Design review of the part built by this model. Coordinates are the model's own, in mm. A direction names the side the tool comes from. Round coordinates to 2 decimals unless told otherwise and drop trailing zeros. Write each loop counter-clockwise with the first axis right and the second up, starting at its lowest first coordinate (ties: lowest second). Pieces come first, ordered by that corner, then holes. Notation, with made-up numbers: M 63.25,89 L 85.25,89 A16 cw 85.25,102 Z; hole C 56,11.25 d1. An arc over 180 degrees is marked long. Use CSV: the item, a comma, the result in double quotes.
from build123d import *

# Parameters (mm, degrees)
SKETCH1_R           = 8
BOSS_EXTRUDE1_DEPTH = 5.8
SKETCH2_R           = 6.5
BOSS_EXTRUDE2_DEPTH = 8
SKETCH3_R           = 6
CUT_EXTRUDE1_DEPTH  = 5.8
SKETCH4_R           = 4.5
CUT_EXTRUDE2_DEPTH  = 7
SKETCH5_R           = 4.5
BOSS_EXTRUDE3_DEPTH = 11
FILLET1_R           = 2


with BuildPart() as part:
    # Sketch1 → Boss-Extrude1 (new body)
    with BuildSketch(Plane(origin=(0, 0, 0), x_dir=(1, 0, 0), z_dir=(0, 1, 0))):
        with Locations(Location((0, 0, 0), (0, 0, 270))):
            Circle(SKETCH1_R)
    extrude(amount=BOSS_EXTRUDE1_DEPTH)

    # Sketch2 → Boss-Extrude2 (add)
    with BuildSketch(Plane(origin=(0, 5.8, 0), x_dir=(-1, 0, 0), z_dir=(0, 1, 0))):
        with Locations(Location((0, 0, 0), (0, 0, 90))):
            Circle(SKETCH2_R)
    extrude(amount=BOSS_EXTRUDE2_DEPTH)

    # Sketch3 → Cut-Extrude1 (cut)
    with BuildSketch(Plane.XZ):
        with Locations(Location((0, 0, 0), (0, 0, 270))):
            Circle(SKETCH3_R)
    extrude(amount=-CUT_EXTRUDE1_DEPTH, mode=Mode.SUBTRACT)

    # Sketch4 → Cut-Extrude2 (cut)
    with BuildSketch(Plane.XZ.offset(-5.8)):
        with Locations(Location((0, 0, 0), (0, 0, 270))):
            Circle(SKETCH4_R)
    extrude(amount=-CUT_EXTRUDE2_DEPTH, mode=Mode.SUBTRACT)

    # Sketch5 → Boss-Extrude3 (add)
    with BuildSketch(Plane(origin=(0, 13.8, 0), x_dir=(-1, 0, 0), z_dir=(0, 1, 0))):
        with Locations(Location((0, 0, 0), (0, 0, 270))):
            Circle(SKETCH5_R)
    extrude(amount=BOSS_EXTRUDE3_DEPTH)

    # Fillet1
    # the kernel refuses this fillet: 2 mm, written as the material it adds along each edge
    with BuildSketch(Plane(origin=(0, 5.8, 0), x_dir=(0, 0, 1), z_dir=(-1, 0, 0))) as fillet1_piece_1:
        with BuildLine():
            CenterArc((8.5, 1.936491673), FILLET1_R, 180, 75.522487814)
            Line((6.5, 1.936491673), (6.5, 0))
            Line((6.5, 0), (8, 0))
        make_face()
    revolve(axis=Axis((0, 5.8, 0), (0, 1, 0)))
    # the kernel refuses this fillet: 2 mm, written as the material it takes off along each edge
    with BuildSketch(Plane(origin=(0, 13.8, 0), x_dir=(0, 0, 1), z_dir=(-1, 0, 0))) as fillet1_2_piece_1:
        with BuildLine():
            CenterArc((6.5 - FILLET1_R, -FILLET1_R), FILLET1_R, 0, 90)
            Line((6.5 - FILLET1_R, 0), (6.5, 0))
            Line((6.5, 0), (6.5, -FILLET1_R))
        make_face()
    revolve(axis=Axis((0, 13.8, 0), (0, 1, 0)), mode=Mode.SUBTRACT)


solid = part.part
1) Add section B-B on y = 3. Write out the cut boundary in (x, z), then the cut area to 3 significant figures.
Answers:
outline,"C 0,0 d16; hole C 0,0 d12"
area,"88.0 mm²"
2) Add section D-D on y = 18.25. Write out the cut boundary in (x, z), then the cut area to 3 significant figures.
Answers:
outline,"C 0,0 d9"
area,"63.6 mm²"
3) Machinability: for faces 1 (the face through (0, 12.8, 0)), 2 (the face through (0, 24.8, 0)), 3 (the face through (-1.352, 19.223, -4.292)), which of the approach directions +Z, -Z, +X, -X, +Y, -Y give a long, thin tool a straight path to every point of the face, cutting with its end or side? Answer none if there is none.
Answers:
face 1,"-Y"
face 2,"+Z, -Z, +X, -X, +Y"
face 3,"+Y"
4) The part is to be moulded in two halves that separate along Z. For faces 4 (the face through (4.5, 5.8, 1.4)), 5 (the face through (6, 0, -2)), 6 (the face through (-7.81, 2.86, -1.73)), say which applies: released by +Z, released by -Z, zero draft, split by the parting line, or undercut.
Answers:
face 4,"undercut"
face 5,"zero draft"
face 6,"split by the parting line"
5) Add section A-A on z = 0. Write out the cut boundary in (x, y).
Answers:
outline,"M -8,0 L -6,0 L -6,5.8 L -4.5,5.8 L -4.5,12.8 L 4.5,12.8 L 4.5,5.8 L 6,5.8 L 6,0 L 8,0 L 8,5.8 A2 cw 6.5,7.74 L 6.5,11.8 A2 ccw 4.5,13.8 L 4.5,24.8 L -4.5,24.8 L -4.5,13.8 A2 ccw -6.5,11.8 L -6.5,7.74 A2 cw -8,5.8 Z"
6) For pin 1 Ø1.5 at (x, z) = (1.5, 4.5) entering from -Y; pin 2 Ø1 at (y, z) = (12.5, 4) entering from -X; pin 3 Ø8 at (x, y) = (-3.5, 10) entering from -Z, all flat-tipped, find the tip position at first contact; note any pin that passes through.
Answers:
pin 1,"y = 5.8"
pin 2,"x = -5.37"
pin 3,"z = -6.87"
7) Add section C-C on x = 0. Write out the cut boundary in (y, z), then the cut area to 3 significant figures.
Answers:
outline,"M 0,-8 L 5.8,-8 A2 cw 7.74,-6.5 L 11.8,-6.5 A2 ccw 13.8,-4.5 L 24.8,-4.5 L 24.8,4.5 L 13.8,4.5 A2 ccw 11.8,6.5 L 7.74,6.5 A2 cw 5.8,8 L 0,8 L 0,6 L 5.8,6 L 5.8,4.5 L 12.8,4.5 L 12.8,-4.5 L 5.8,-4.5 L 5.8,-6 L 0,-6 Z"
area,"163 mm²"
8) Wall thickness on line 1 along X through (y, z) = (1.7, 0); line 2 along X through (y, z) = (16.5, 0.25); line 3 along Y through (x, z) = (-3, 0.75): over which ranges is each line inside the solid? List them lowest first. Write a range as [from, to].
Answers:
line 1,"[-8, -6], [6, 8]"
line 2,"[-4.49, 4.49]"
line 3,"[12.8, 24.8]"
